Geometry check sheet. Reference: the model listing, model coordinates, mm. Face numbers are marked on the shaded views. A direction names the side the tool comes from. Give positions to 0.01 mm unless a question says otherwise; leave off trailing zeros. Loops run counter-clockwise (first coordinate to the right, second up) from the corner with the lowest first, then second, coordinate; pieces in that order, holes last. Notation, with made-up numbers: (-20, 82.5) -> (-2, 82.5) arc R26 ccw to (-2, 100.5) -> close; hole circle Ø8 at (12, 66). An arc over 180 degrees is marked (long way). Answer as a JSON object with one key per item and string values.
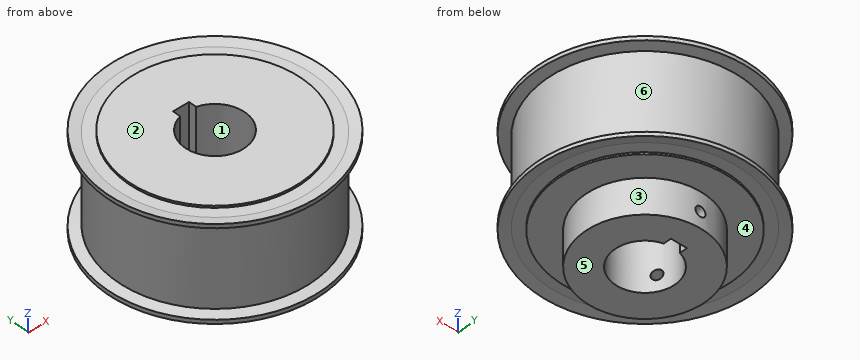
from build123d import *

# Parameters (mm, degrees)
SKETCH2_W                  = 65
SKETCH2_H                  = 15
CUT_EXTRUDE1_DEPTH         = 101.284595028
M6X1_0_TAPPED_HOLE1_REACH  = 147.812
M6X1_0_TAPPED_HOLE1_BORE_R = 2.5
CIRPATTERN1_COUNT          = 2
CIRPATTERN1_ANGLE          = 120


with BuildPart() as part:
    # Sketch1 → Revolve1 (revolve)
    with BuildSketch(Plane(origin=(0, 0, 0), x_dir=(0, 0, -1), z_dir=(1, 0, 0)), mode=Mode.PRIVATE) as revolve1_sk:
        Polygon((-65, 43.5), (-64, 43.5), (-64, 48.965), (-65, 54), (-63, 54), (-62, 48.965), (-20.5, 48.965), (-19.5, 54), (-17.5, 54), (-18.5, 48.965), (-18.5, 43.5), (-17.5, 43.5), (-17.5, 30), (0, 30), (0, 0), (-65, 0), align=None)
    revolve(revolve1_sk.sketch.rotate(Axis((0, 0, 66.142918398), (0, 0, -1)), 90), axis=Axis((0, 0, 66.142918398), (0, 0, -1)))

    # Sketch2 → Cut-Revolve1 (revolve, cut)
    with BuildSketch(Plane(origin=(0, 0, 0), x_dir=(0, 0, -1), z_dir=(1, 0, 0)), mode=Mode.PRIVATE) as cut_revolve1_sk:
        with Locations((-32.5, 7.5)):
            Rectangle(SKETCH2_W, SKETCH2_H)
    revolve(cut_revolve1_sk.sketch.rotate(Axis((0, 0, -15.356501925), (0, 0, 1)), 90), axis=Axis((0, 0, -15.356501925), (0, 0, 1)), mode=Mode.SUBTRACT)

    # Sketch3 → Cut-Extrude1 (cut, through all)
    with BuildSketch(Plane.XY.offset(65)):
        with BuildLine():
            Line((-4, 18.3), (4, 18.3))
            Line((4, 18.3), (4, 14.456832295))
            ThreePointArc((4, 14.456832295), (0, 15), (-4, 14.456832295))
            Line((-4, 14.456832295), (-4, 18.3))
        make_face()
    extrude(amount=-CUT_EXTRUDE1_DEPTH, mode=Mode.SUBTRACT)

    # M6x1.0 Tapped Hole1 bore → M6x1.0 Tapped Hole1 (cut, up to next)
    with BuildSketch(Plane(origin=(0, 30, -41.25), x_dir=(-1, 0, 0), z_dir=(0, 1, 0)), mode=Mode.PRIVATE) as m6x1_0_tapped_hole1_sk1:
        with Locations((0, 49.25)):
            Circle(M6X1_0_TAPPED_HOLE1_BORE_R)
    m6x1_0_tapped_hole1_tool1 = extrude(m6x1_0_tapped_hole1_sk1.sketch, amount=-M6X1_0_TAPPED_HOLE1_REACH, mode=Mode.PRIVATE) & part.part
    m6x1_0_tapped_hole1 = m6x1_0_tapped_hole1_tool1.solids().sort_by_distance((0, 30, 8))[0]
    add(m6x1_0_tapped_hole1, mode=Mode.SUBTRACT)

    # CirPattern1: M6x1.0 Tapped Hole1; each copy of M6x1.0 Tapped Hole1 runs up to whatever stops it at its own place
    cirpattern1_before = part.part  # the part as the pattern finds it: every copy runs up to it
    cirpattern1_m6x1_0_tapped_hole1_long = extrude(m6x1_0_tapped_hole1_sk1.sketch, amount=-M6X1_0_TAPPED_HOLE1_REACH, mode=Mode.PRIVATE)
    cirpattern1_m6x1_0_tapped_hole1_tool1 = cirpattern1_m6x1_0_tapped_hole1_long.rotate(Axis((0, 0, -15.356501925), (0, 0, 1)), 1 * CIRPATTERN1_ANGLE / (CIRPATTERN1_COUNT - 1)) & cirpattern1_before
    add(cirpattern1_m6x1_0_tapped_hole1_tool1.solids().sort_by_distance((-25.980762, -15, 8))[0], mode=Mode.SUBTRACT)


solid = part.part
1) Tool access check on the marked faces 4, 5 and 6. Record the directions out of +Z, -Z, +X, -X, +Y, -Y that give a thin tool (end or side, any length) a straight path to the whole face; none if there is none.
Geometry check:
{"face 4": "-Z", "face 5": "-Z, +X, -X, +Y, -Y", "face 6": "none"}
2) Depth check by flat-ended pin: P1, Ø1.5, axis at y = -17.5, z = 15.5, coming from the -X side; P2, Ø8, axis at x = 0, z = 8, coming from the -Y side; P3, Ø10, axis at x = 28.5, z = 54, coming from the +Y side. Enter the tip coordinate at first touch or a pass-through.
Geometry check:
{"P1": "stops at x = -24.89", "P2": "stops at y = -30", "P3": "stops at y = 42.96"}
3) Section check C-C on z = 52. Record the cut outline in (x, y) (3 decimals).
Geometry check:
{"outline": "circle Ø97.93 at (0, 0); hole (-4, 14.457) arc R15 ccw (long way) to (4, 14.457) -> (4, 18.3) -> (-4, 18.3) -> close"}
4) Section check D-D on z = 8. Record the cut outline in (x, y), plus the area to 3 significant figures.
Geometry check:
{"outline": "(-27.14, -12.78) -> (-14.06, -5.23) arc R15 cw to (-4, 14.46) -> (-4, 18.3) -> (-2.5, 18.3) -> (-2.5, 29.9) arc R30 ccw to start; (-24.64, -17.11) arc R30 ccw (long way) to (2.5, 29.9) -> (2.5, 18.3) -> (4, 18.3) -> (4, 14.46) arc R15 cw (long way) to (-11.56, -9.56) -> close", "area": "1,960 mm2"}
5) Draft check along X on the marked faces 1, 2 and 3. Enter one of: pulls with the +X half, pulls with the -X half, needs draft (parallel to the pull), parting line crosses it, or undercut.
Geometry check:
{"face 1": "undercut", "face 2": "needs draft", "face 3": "parting line crosses it"}
6) Material ranges on line 1 along Z through (x, y) = (0, 22.25); line 2 along Z through (x, y) = (-38.5, 25.5); line 3 along X through (y, z) = (22, 8), recorded low to high. Write a range as from..to.
Geometry check:
{"line 1": "z = 0..5.5, 10.5..65", "line 2": "z = 18.5..64", "line 3": "x = -20.4..-2.5, 2.5..20.4"}
7) Section check B-B on x = 0. Count the separate pieces of the cut face and the enclosed holes in it, plus the area to 3 significant figures.
Geometry check:
{"separate pieces": "3", "enclosed holes": "0", "area": "3,500 mm2"}
